Read the model definition and answer for the solid it produces. Units are mm, in the model's axes. Give positions to 0.01 mm unless a question says otherwise; leave off trailing zeros. Order: outer loops, then holes, each group sorted by start corner. A loop starts at its lowest first (then second) coordinate and runs counter-clockwise, first axis right, second up.
Item 1: A cutting plane is placed at A-A (y = 90). Write down the section's boundary in (x, z), plus the area to 3 significant figures.
Item 2: Given pin 1 Ø4 at (x, y) = (0, -30) entering from -Z, flat-ended and moving along its own axis, determine where the tip first touches the part or whether it passes through.
Item 3: A cutting plane is placed at B-B (x = -33). Write down the section's boundary in (y, z).
Item 4: A cutting plane is placed at C-C (z = 3.05). State how many separate pieces and enclosed holes the cut face has, plus the area to 3 significant figures.
Item 5: Find the intervals of material crossed by line 1 along X through (y, z) = (-135, 3.15); line 2 along X through (y, z) = (-113, 0.55); line 3 along X through (y, z) = (27, 1.9), in increasing order.
from build123d import *

# Parameters (mm, degrees)
SKETCH_1_W          = 170
SKETCH_1_H          = 290
EXTRUDE_1_DEPTH     = 5
SKETCH_2_R          = 13.5
CUT_EXTRUDE_1_DEPTH = 169.151717208
SKETCH_3_R          = 2.5
CUT_EXTRUDE_2_DEPTH = 169.151717208
CHAMFER_1_SIZE      = 10
SKETCH_4_R          = 7.5
SKETCH_4_R_2        = 2.5
CUT_EXTRUDE_3_DEPTH = 169.151717208
CUT_EXTRUDE_4_DEPTH = 169.151717208
FILLET_1_R          = 10


with BuildPart() as part:
    # ｽｹｯﾁ1 → ﾎﾞｽ - 押し出し1 (new body)
    with BuildSketch(Plane.XY):
        Rectangle(SKETCH_1_W, SKETCH_1_H)
    extrude(amount=EXTRUDE_1_DEPTH)

    # ｽｹｯﾁ2 → ｶｯﾄ - 押し出し1 (cut, through all)
    with BuildSketch(Plane.XY.offset(5)):
        Circle(SKETCH_2_R)
    extrude(amount=-CUT_EXTRUDE_1_DEPTH, mode=Mode.SUBTRACT)

    # ｽｹｯﾁ3 → ｶｯﾄ - 押し出し2 (cut, through all)
    with BuildSketch(Plane.XY.offset(5)):
        with Locations((-75, 0)):
            Circle(SKETCH_3_R)
        with Locations((0, 135)):
            Circle(SKETCH_3_R)
        with Locations((75, 0)):
            Circle(SKETCH_3_R)
        with Locations((0, -135)):
            Circle(SKETCH_3_R)
        with Locations((-60, 135)):
            Circle(SKETCH_3_R)
        with Locations((60, 135)):
            Circle(SKETCH_3_R)
        with Locations((60, -135)):
            Circle(SKETCH_3_R)
        with Locations((-60, -135)):
            Circle(SKETCH_3_R)
    extrude(amount=-CUT_EXTRUDE_2_DEPTH, mode=Mode.SUBTRACT)

    # 面取り1
    chamfer_1_edges = [part.edges().sort_by_distance(p)[0] for p in [
        (85, -145, 2.5),
        (-85, -145, 2.5),
        (-85, 145, 2.5),
        (85, 145, 2.5),
    ]]
    chamfer(chamfer_1_edges, length=CHAMFER_1_SIZE)

    # ｽｹｯﾁ4 → ｶｯﾄ - 押し出し3 (cut, through all)
    with BuildSketch(Plane.XY.offset(5)):
        with Locations((90, 90)):
            Circle(SKETCH_4_R)
        with Locations((0, 90)):
            Circle(SKETCH_4_R)
        with Locations((-90, 90)):
            Circle(SKETCH_4_R)
        with Locations((-90, -90)):
            Circle(SKETCH_4_R)
        with Locations(Location((0, -90, 0), (0, 0, 180))):
            Circle(SKETCH_4_R)
        with Locations((90, -90)):
            Circle(SKETCH_4_R)
        with Locations((0, -30)):
            Circle(SKETCH_4_R_2)
        with Locations((-25.980762114, -15)):
            Circle(SKETCH_4_R_2)
        with Locations((-25.980762114, 15)):
            Circle(SKETCH_4_R_2)
        with Locations((0, 30)):
            Circle(SKETCH_4_R_2)
        with Locations((25.980762114, 15)):
            Circle(SKETCH_4_R_2)
        with Locations((25.980762114, -15)):
            Circle(SKETCH_4_R_2)
    extrude(amount=-CUT_EXTRUDE_3_DEPTH, mode=Mode.SUBTRACT)

    # ｽｹｯﾁ5 → ｶｯﾄ - 押し出し4 (cut, through all)
    with BuildSketch(Plane.XY.offset(5)):
        with BuildLine():
            Line((-65, 125), (-65, 15))
            Line((-65, 15), (-42.426406871, 15))
            ThreePointArc((-42.426406871, 15), (-31.819805153, 31.819805153), (-15, 42.426406871))
            Line((-15, 42.426406871), (-15, 125))
            Line((-15, 125), (-65, 125))
        make_face()
        with BuildLine():
            Line((15, 42.426406871), (15, 125))
            Line((15, 125), (65, 125))
            Line((65, 125), (65, 15))
            Line((65, 15), (42.426406871, 15))
            ThreePointArc((42.426406871, 15), (31.819805153, 31.819805153), (15, 42.426406871))
        make_face()
        with BuildLine():
            Line((-15, -42.426406871), (-15, -125))
            Line((-15, -125), (-65, -125))
            Line((-65, -125), (-65, -15))
            Line((-65, -15), (-42.426406871, -15))
            ThreePointArc((-42.426406871, -15), (-31.819805153, -31.819805153), (-15, -42.426406871))
        make_face()
        with BuildLine():
            Line((15, -42.426406871), (15, -125))
            Line((15, -125), (65, -125))
            Line((65, -125), (65, -15))
            Line((65, -15), (42.426406871, -15))
            ThreePointArc((42.426406871, -15), (31.819805153, -31.819805153), (15, -42.426406871))
        make_face()
    extrude(amount=-CUT_EXTRUDE_4_DEPTH, mode=Mode.SUBTRACT)

    # ﾌｨﾚｯﾄ1
    fillet_1_edges = [part.edges().sort_by_distance(p)[0] for p in [
        (42.426406871, 15, 2.5),
        (15, 42.426406871, 2.5),
        (15, 125, 2.5),
        (65, 125, 2.5),
        (65, 15, 2.5),
        (-42.426406871, -15, 2.5),
        (-15, -42.426406871, 2.5),
        (-15, -125, 2.5),
        (-65, -125, 2.5),
        (-65, -15, 2.5),
        (15, -42.426406871, 2.5),
        (42.426406871, -15, 2.5),
        (65, -15, 2.5),
        (65, -125, 2.5),
        (15, -125, 2.5),
        (-65, 125, 2.5),
        (-15, 125, 2.5),
        (-15, 42.426406871, 2.5),
        (-42.426406871, 15, 2.5),
        (-65, 15, 2.5),
    ]]
    fillet(fillet_1_edges, radius=FILLET_1_R)


solid = part.part
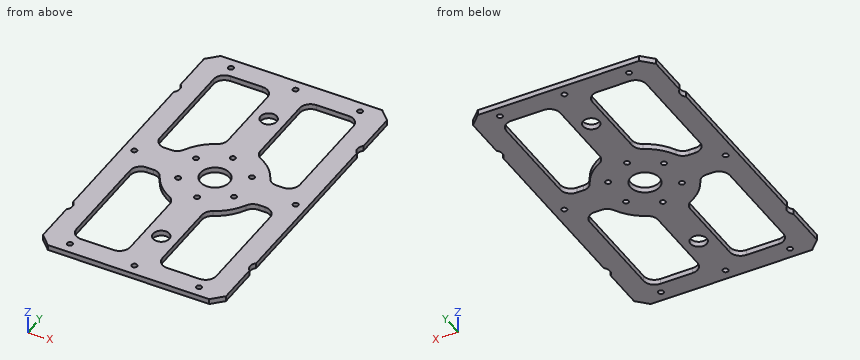
Response values:
1. outline: (-82.5, 0) - (-65, 0) - (-65, 5) - (-82.5, 5) - close; (-15, 0) - (-7.5, 0) - (-7.5, 5) - (-15, 5) - close; (7.5, 0) - (15, 0) - (15, 5) - (7.5, 5) - close; (65, 0) - (82.5, 0) - (82.5, 5) - (65, 5) - close
1. area: 250 mm2
2. pin 1: passes through
3. outline: (-145, 0) - (-125, 0) - (-125, 5) - (-145, 5) - close; (-30.59, 0) - (30.59, 0) - (30.59, 5) - (-30.59, 5) - close; (125, 0) - (145, 0) - (145, 5) - (125, 5) - close
4. separate pieces: 1
4. enclosed holes: 21
4. area: 28,100 mm2
5. line 1: x = -85 to -62.5, -57.5 to -2.5, 2.5 to 57.5, 62.5 to 85
5. line 2: x = -85 to -65, -15 to 15, 65 to 85
5. line 3: x = -85 to -65, -36 to 36, 65 to 85
